Verification items for the finished model (mm, model axes). Face numbers are marked on the shaded views. A direction names the side the tool comes from. Coordinates: 2 decimals unless noted, no trailing zeros. Order: outer loops, then holes, each group sorted by start corner. A loop starts at its lowest first (then second) coordinate and runs counter-clockwise, first axis right, second up. Notation, with made-up numbers: (19.5, -37) - (26.5, -37) arc R28 ccw to (26.5, 0) - close; hole circle Ø5 at (-11.5, 55). An arc over 180 degrees is marked (long way). Answer as CSV lines item,"result". Start each with the question number.
1. Set-up check for the marked faces 1 and 2: record each of +Z, -Z, +X, -X, +Y, -Y from which the full face is reachable in a straight line by a thin tool's end or side.
2. Section check A-A (x = 15). Record the cut outline in (y, z), and give its area (3 significant figures).
3. Material ranges on L1, parallel to X at y = 288, z = -4.25; L2, parallel to Y at x = -12, z = 6.25; L3, parallel to Y at x = -11.5, z = -2, recorded low to high. Write a range as [from, to].
4. Section check B-B (y = 116.5). Record the cut outline in (x, z).
5. Section check C-C (z = -5). Record the cut outline in (x, y), and give its area (3 significant figures).
6. Mould release check, pull along X, two halves, no side actions. Record for the marked faces 3 and 4: pulls with the +X half, pulls with the -X half, needs draft (parallel to the pull), parting line crosses it, or undercut.
7. Go/stop test with flat-tipped pins: pin 1 (1 mm diameter, centred on x = 39, z = 4, fed in from +Y); pin 2 (5 mm diameter, centred on x = 33, z = -3.5, fed in from -Y). Record where each tip stops, or that it passes through.
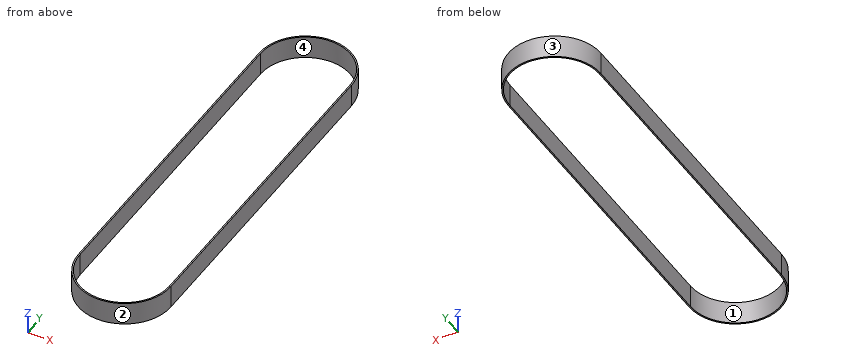
Autodesk Inventor part; units mm, degrees
ref_plane "Cross Section Plane" through (-16.831, 296.54, 0) normal (0, -1, 0) x (0, 0, 1)
ref_plane "Work Plane2" through (15, 296.54, 0) normal (-1, 0, 0) x (0, 0, 1)
ref_plane "Work Plane3" through (15, 71.54, 0) normal (0.1564, 0.9877, 0) x (0, 0, 1)
sketch "Sketch Path" plane through (0, 0, 0) normal (0, 0, 1) x (1, 0, 0)
  arc A0 (46.831, 296.54) -> (-16.831, 296.54) centre (15, 296.54) ccw
  arc A1 (-16.831, 71.54) -> (46.831, 71.54) centre (15, 71.54) ccw
  line L0 (-16.831, 71.54) -> (-16.831, 296.54)
  line L1 (46.831, 296.54) -> (46.831, 71.54)
ref_plane "Cross Section Plane" through (-16.831, 296.54, 0) normal (0, -1, 0) x (0, 0, 1)
ref_plane "Work Plane2" through (15, 296.54, 0) normal (-1, 0, 0) x (0, 0, 1)
ref_plane "Work Plane3" through (15, 71.54, 0) normal (0.1564, 0.9877, 0) x (0, 0, 1)
sketch "Cross Section" plane through (-16.831, 296.54, 0) normal (0, -1, 0) x (0, 0, 1)
  line L0 (-8, 0.5) -> (8, 0.5)
  line L1 (8, 0.5) -> (8, -0.5)
  line L2 (8, -0.5) -> (-8, -0.5)
  line L3 (-8, -0.5) -> (-8, 0.5)
  line L4 (-8, 0) -> (8, 0) construction
  point P0 (0, 0)
  point P1 (0, 0)
  dimension "d0" = 16
  dimension "d4" = 0.5
  dimension "d5" = 0.5
sweep "Belt" add profiles "Cross Section" path "Sketch Path"
equation "\"d0\" = da_B"
equation "\"d4\" = da_a"
equation "\"d5\" = da_a2"
equation "\"da_B\" = 16"
equation "\"da_pb\" = 5"
equation "\"da_a\" = 0.5"
equation "\"da_S\" = 2.65"
equation "\"da_Beta\" = 20deg"
equation "\"da_Ht\" = 1.2"
equation "\"da_H\" = 3.4"
equation "\"da_a2\" = 0.5"
properties part number "Synchronous Belt" material "Rubber"
Evaluation:
1,face 1,"+Z, -Z"
1,face 2,"+Z, -Z, -Y"
2,outline,"(39.21, -8) - (40.21, -8) - (40.21, 8) - (39.21, 8) - close; (327.87, -8) - (328.87, -8) - (328.87, 8) - (327.87, 8) - close"
2,area,"32.0 mm²"
3,L1,"x = [-17.33, -16.33], [46.33, 47.33]"
3,L2,"y = [53.76, 55.65], [312.43, 314.32]"
3,L3,"y = [53.02, 54.83], [313.25, 315.06]"
4,outline,"(-17.33, -8) - (-16.33, -8) - (-16.33, 8) - (-17.33, 8) - close; (46.33, -8) - (47.33, -8) - (47.33, 8) - (46.33, 8) - close"
5,outline,"(-17.33, 71.54) arc R32.33 ccw to (47.33, 71.54) - (47.33, 296.54) arc R32.33 ccw to (-17.33, 296.54) - close; hole (-16.33, 71.54) arc R31.33 ccw to (46.33, 71.54) - (46.33, 296.54) arc R31.33 ccw to (-16.33, 296.54) - close"
5,area,"650 mm²"
6,face 3,"parting line crosses it"
6,face 4,"undercut"
7,pin 1,"stops at y = 318.74"
7,pin 2,"stops at y = 43.17"
